from build123d import *

# Parameters (mm, degrees)
F0_R     = 304.8
F1_DEPTH = 19.05
F4_W     = 651.788891
F4_H     = 160.561264
F5_DEPTH = 25.4


with BuildPart() as f1:
    # F0 (on Top) → F1 (new body)
    with BuildSketch(Plane.XY):
        Circle(F0_R)
    extrude(amount=F1_DEPTH)

    # F4 (on face) → F5 (cut)
    with BuildSketch(Plane.XY.offset(19.05)):
        with Locations((-6.526291, -280.289799)):
            Rectangle(F4_W, F4_H)
        with Locations((-6.526291, 280.289799)):
            Rectangle(F4_W, F4_H)
    extrude(amount=-F5_DEPTH, mode=Mode.SUBTRACT)


with BuildPart() as f2_1:
    # F2: copy of F1
    add(f1.part.moved(Location((0, 0, -515.62))))


solid = f1.part
Model file for the job. Use its own axes, mm. Give positions to 0.01 mm unless a question says otherwise; leave off trailing zeros. Order: outer loops, then holes, each group sorted by start corner. A loop starts at its lowest first (then second) coordinate and runs counter-clockwise, first axis right, second up. Notation, with made-up numbers: (-34, -4) - (11, -4) arc R22 cw to (11, 19) - close; hole circle Ø1 at (-30.5, 27). An arc over 180 degrees is marked (long way). One line per item, written item: value.
Item 1: Wall check: line 1 (X direction, y = 49.5, z = 7); line 2 (X direction, y = -47, z = 10.25); line 3 (Y direction, x = 231.5, z = 10.5). Give the ranges that are in metal, low to high.
Response values:
line 1: -300.75 to 300.75
line 2: -301.15 to 301.15
line 3: -198.27 to 198.27
Item 2: Slice it at B-B (y = -129.5). List the corners of the cut face in (x, z), then the cut area to 3 significant figures.
Response values:
outline: (-275.92, 0) - (275.92, 0) - (275.92, 19.05) - (-275.92, 19.05) - close
area: 10,500 mm2
Item 3: Pin check, flat tips, straight feed: pin 1 Ø8 at (y, z) = (-142.5, 4.5) entering from +X; pin 2 Ø2 at (y, z) = (141.5, 12) entering from -X; pin 3 Ø5 at (y, z) = (125.5, 11) entering from -X. Stop position of each tip, or through.
Response values:
pin 1: x = 271.52
pin 2: x = -270.49
pin 3: x = -278.88
Item 4: Slice it at A-A (z = 4.25). List the corners of the cut face in (x, y).
Response values:
outline: (-230, -200.01) - (230, -200.01) arc R304.8 ccw to (230, 200.01) - (-230, 200.01) arc R304.8 ccw to start
